```python
from build123d import *

# Parameters (mm, degrees)
F0_R     = 3.2766
F1_DEPTH = 8.89
F2_R     = 4.699
F3_DEPTH = 1.778
F4_R     = 2.7305
F5_DEPTH = 3.81
F6_R     = 3.2766
F6_R_2   = 1.6891
F7_DEPTH = 13.462


with BuildPart() as f1:
    # F0 (on Top) → F1 (new body)
    with BuildSketch(Plane.XY):
        Circle(F0_R)
    extrude(amount=F1_DEPTH)

    # F2 (on Top) → F3 (join)
    with BuildSketch(Plane.XY):
        Circle(F2_R)
    extrude(amount=F3_DEPTH)

    # F4 (on face) → F5 (join)
    with BuildSketch(Plane(origin=(0, 0, 0), x_dir=(1, 0, 0), z_dir=(0, 0, -1))):
        Circle(F4_R)
    extrude(amount=F5_DEPTH)

    # F6 (on face) → F7 (join)
    with BuildSketch(Plane.XY.offset(8.89)):
        Circle(F6_R)
        Circle(F6_R_2, mode=Mode.SUBTRACT)
    extrude(amount=F7_DEPTH)


solid = f1.part
```
Verification items for the finished model (mm, model axes). A direction names the side the tool comes from. Give positions to 0.01 mm unless a question says otherwise; leave off trailing zeros. Order: outer loops, then holes, each group sorted by start corner. A loop starts at its lowest first (then second) coordinate and runs counter-clockwise, first axis right, second up. Notation, with made-up numbers: (87.25, 36.25) -> (135.25, 36.25) arc R22 cw to (135.25, 63.25) -> close; hole circle Ø6 at (59.5, 72). An arc over 180 degrees is marked (long way). Use a Markdown table: item, result.
1) Mould release check, pull along X, two halves, no side actions. Record for faces 4 (the cylindrical face through (2.604, -0.82, -1.878)), 5 (the flat face through (0, 0, 8.89)), 6 (the cylindrical face through (-1.34, -1.03, 15.53)), 7 (the flat face through (0, 0, -3.81)): pulls with the +X half, pulls with the -X half, needs draft (parallel to the pull), parting line crosses it, or undercut.
Results:
| item | result |
|---|---|
| face 4 | parting line crosses it |
| face 5 | undercut |
| face 6 | undercut |
| face 7 | needs draft |
2) Section check D-D, the plane y = -3. Record the boundary of the cut face in (x, z).
Results:
| item | result |
|---|---|
| outline | (-3.62, 0) -> (3.62, 0) -> (3.62, 1.78) -> (1.32, 1.78) -> (1.32, 22.35) -> (-1.32, 22.35) -> (-1.32, 1.78) -> (-3.62, 1.78) -> close |
3) Material ranges on probe 1 along Y at (x, z) = (0, 15.75); probe 2 along X at (y, z) = (0, 2.5); probe 3 along Z at (x, y) = (4, 0), recorded low to high.
Results:
| item | result |
|---|---|
| probe 1 | -3.28 to -1.69, 1.69 to 3.28 |
| probe 2 | -3.28 to 3.28 |
| probe 3 | 0 to 1.78 |
4) Section check A-A, the plane x = 0. Record the boundary of the cut face in (y, z), then the cut area to 3 significant figures.
Results:
| item | result |
|---|---|
| outline | (-4.7, 0) -> (-2.73, 0) -> (-2.73, -3.81) -> (2.73, -3.81) -> (2.73, 0) -> (4.7, 0) -> (4.7, 1.78) -> (3.28, 1.78) -> (3.28, 22.35) -> (1.69, 22.35) -> (1.69, 8.89) -> (-1.69, 8.89) -> (-1.69, 22.35) -> (-3.28, 22.35) -> (-3.28, 1.78) -> (-4.7, 1.78) -> close |
| area | 127 mm² |
5) Depth check by flat-ended pin: pin 1 Ø1 at (x, z) = (-2.5, 10) entering from +Y; pin 2 Ø1.5 at (x, z) = (2, 2) entering from +Y; pin 3 Ø1.5 at (y, z) = (2, 8.5) entering from +X. Enter the tip coordinate at first touch or a pass-through.
Results:
| item | result |
|---|---|
| pin 1 | y = 2.6 |
| pin 2 | y = 4.52 |
| pin 3 | x = 3.03 |
6) Tool access check on faces 1 (the flat face through (0, -3, 0)), 2 (the flat face through (-2, 1, 22.352)), 3 (the cylindrical face through (-2.415, 2.214, 11.921)). Record the directions out of +Z, -Z, +X, -X, +Y, -Y that give a thin tool (end or side, any length) a straight path to the whole face; none if there is none.
Results:
| item | result |
|---|---|
| face 1 | -Z |
| face 2 | +Z, +X, -X, +Y, -Y |
| face 3 | +Z |
7) Section check C-C, the plane z = 15.75. Record the boundary of the cut face in (x, y), then the cut area to 3 significant figures.
Results:
| item | result |
|---|---|
| outline | circle Ø6.55 at (0, 0); hole circle Ø3.38 at (0, 0) |
| area | 24.8 mm² |
